Autodesk Inventor part; units mm, degrees
ref_plane "YZ Plane" through (0, 0, 0) normal (1, 0, 0) x (0, 1, 0)
ref_plane "XZ Plane" through (0, 0, 0) normal (0, 1, 0) x (-1, 0, 0)
ref_plane "XY Plane" through (0, 0, 0) normal (0, 0, 1) x (1, 0, 0)
sketch "Sketch1" plane through (0, 0, 0) normal (0, 0, 1) x (1, 0, 0)
  line L0 (-130, -50) -> (130, -50)
  line L1 (130, -50) -> (130, 50)
  line L2 (130, 50) -> (-130, 50)
  line L3 (-130, 50) -> (-130, -50)
  line L4 (-130, -50) -> (130, 50) construction
  line L5 (130, -50) -> (-130, 50) construction
  line L6 (-75, -50) -> (-25, -50)
  line L7 (-25, -50) -> (-25, -55)
  line L8 (-25, -55) -> (-75, -55)
  line L9 (-75, -55) -> (-75, -50)
  line L10 (25, -50) -> (75, -50)
  line L11 (75, -50) -> (75, -55)
  line L12 (75, -55) -> (25, -55)
  line L13 (25, -55) -> (25, -50)
  line L14 (130, 50) -> (125, 50)
  line L15 (125, 50) -> (125, 30)
  line L16 (125, 30) -> (130, 30)
  line L17 (130, 30) -> (130, 50)
  line L18 (130, -50) -> (125, -50)
  line L19 (125, -50) -> (125, -30)
  line L20 (125, -30) -> (130, -30)
  line L21 (130, -30) -> (130, -50)
  line L22 (0, 50) -> (0, -50) construction
  line L23 (-125, 50) -> (-125, 30)
  line L24 (-125, 30) -> (-130, 30)
  line L25 (-125, -50) -> (-125, -30)
  line L26 (-125, -30) -> (-130, -30)
  point P0 (0, 0)
  point P1 (-75, -52.5)
  point P2 (75, -50)
  point P3 (-125, -50)
  point P4 (130, -30)
  point P5 (130, 30)
  point P6 (125, 50)
  point P7 (-125, 50)
  point P8 (-130, 30)
  dimension "d0" = 260
  dimension "d1" = 100
  dimension "d2" = 50
  dimension "d3" = 50
  dimension "d4" = 50
  dimension "d5" = 55
  dimension "d6" = 5
  dimension "d10" = 20
  dimension "d12" = 5
  dimension "d13" = 20
extrude "Extrusion1" add sketch "Sketch1" along normal blind 5 contours L25 L26 L3 L24 L23 L2 L15 L16 L1 L20 L19 L0 | L0 L7 L8 L9 | L0 L11 L12 L13
equation "\"BendRadius\" = Thickness"
equation "\"BendReliefWidth\" = Thickness"
equation "\"BendReliefDepth\" = 0.5 * Thickness"
equation "\"CornerReliefSize\" = 4 * Thickness"
equation "\"MinimumRemnant\" = 2 * Thickness"
equation "\"TransitionRadius\" = BendRadius"
equation "\"JacobiRadiusSize\" = BendRadius"
equation "\"GapSize\" = Thickness"
properties part number "Lat1(3)" material "Wood (Cherry)"
Build history of the part. All positions in model axes, mm. A direction names the side the tool comes from. Coordinates: 2 decimals unless noted, no trailing zeros. Order: outer loops, then holes, each group sorted by start corner. A loop starts at its lowest first (then second) coordinate and runs counter-clockwise, first axis right, second up.
Item 1: Drill centre line: L1, parallel to Y at x = -19, z = 4.05. Where is it in solid material? Low to high.
Filled in:
L1: y = -50 to 50
Item 2: Saw through at C-C on y = 33.5. List the corners of the cut face in (x, z).
Filled in:
outline: (-125, 0) - (125, 0) - (125, 5) - (-125, 5) - close
Item 3: Drop flat-ended pins along their axis: pin 1 Ø2.5 at (x, z) = (-128.5, 2) entering from -Y; pin 2 Ø2.5 at (y, z) = (-52, 3) entering from -X; pin 3 Ø1.5 at (y, z) = (37.5, 2.5) entering from +X; pin 4 Ø12 at (x, y) = (-16.5, 0.5) entering from -Z. Give the stop position or say it passes through.
Filled in:
pin 1: stops at y = -30
pin 2: stops at x = -75
pin 3: stops at x = 125
pin 4: stops at z = 0
Item 4: Tool access for faces 1 (the flat face through (75, -52, 2)), 2 (the flat face through (-127, -30, 2)), 3 (the flat face through (-125, 40, 2)), 4 (the flat face through (-25, -52, 2)): list every direction of +Z, -Z, +X, -X, +Y, -Y with a clear straight run to the whole face (end or side of a thin tool).
Filled in:
face 1: +Z, -Z, +X, -Y
face 2: +Z, -Z, -X, -Y
face 3: +Z, -Z, -X, +Y
face 4: +Z, -Z, -Y
Item 5: Mould opens along X. For faces 5 (the flat face through (25, -53, 2)), 6 (the flat face through (125, 40, 2)), 7 (the flat face through (0, -50, 2)), 8 (the flat face through (-75, -53, 2)) say: released by +X, released by -X, zero draft, split by the parting line, or undercut.
Filled in:
face 5: undercut
face 6: released by +X
face 7: undercut
face 8: released by -X
Item 6: Saw through at A-A on z = 4.1. List the corners of the cut face in (x, y), then the cut area to 3 significant figures.
Filled in:
outline: (-130, -30) - (-125, -30) - (-125, -50) - (-75, -50) - (-75, -55) - (-25, -55) - (-25, -50) - (25, -50) - (25, -55) - (75, -55) - (75, -50) - (125, -50) - (125, -30) - (130, -30) - (130, 30) - (125, 30) - (125, 50) - (-125, 50) - (-125, 30) - (-130, 30) - close
area: 26,100 mm2
Item 7: Saw through at B-B on x = 89.5. List the corners of the cut face in (y, z).
Filled in:
outline: (-50, 0) - (50, 0) - (50, 5) - (-50, 5) - close
